```python
from build123d import *

# Parameters (mm, degrees)
EXTRUDE_THIN1_DEPTH             = 38.1
EXTRUDE1_DEPTH                  = 22.225
EXTRUDE2_REACH                  = 191.48
EXTRUDE2_END_RADIUS             = 58.254302176
SKETCH3_R                       = 14.2875
EXTRUDE2_DIRECTION_2_REACH      = 191.48
EXTRUDE2_DIRECTION_2_END_RADIUS = 36.120408138


with BuildPart() as part:
    # Sketch1 → Extrude-Thin1 (new, symmetric)
    with BuildSketch(Plane.XY):
        with BuildLine():
            Line((0, 0), (47.386965401, 0))
            ThreePointArc((47.386965401, 0), (51.527837673, 1.535887743), (53.665587121, 5.400574229))
            ThreePointArc((53.665587121, 5.400574229), (89.379977527, 36.120408138), (125.094367933, 5.400574229))
            ThreePointArc((125.094367933, 5.400574229), (127.232117381, 1.535887743), (131.372989653, 0))
            Line((131.372989653, 0), (178.759955054, 0))
            Line((178.759955054, 0), (178.759955054, -2.54))
            Line((178.759955054, -2.54), (131.372989653, -2.54))
            ThreePointArc((131.372989653, -2.54), (125.575768472, -0.38975716), (122.582919245, 5.02080392))
            ThreePointArc((122.582919245, 5.02080392), (89.379977527, 33.580408138), (56.177035809, 5.02080392))
            ThreePointArc((56.177035809, 5.02080392), (53.184186582, -0.38975716), (47.386965401, -2.54))
            Line((47.386965401, -2.54), (0, -2.54))
            Line((0, -2.54), (0, 0))
        make_face()
    extrude(amount=EXTRUDE_THIN1_DEPTH, both=True)



with BuildPart() as body_2:
    # Sketch2 → Extrude1 (new, symmetric)
    with BuildSketch(Plane.XY):
        with BuildLine():
            Line((69.175001958, 75.045019307), (109.584953096, 75.045019307))
            Line((109.584953096, 75.045019307), (109.584953096, 65.256940868))
            ThreePointArc((109.584953096, 65.256940868), (89.379977527, 61.640745213), (69.175001958, 65.256940868))
            Line((69.175001958, 65.256940868), (69.175001958, 75.045019307))
        make_face()
    extrude(amount=EXTRUDE1_DEPTH, both=True)


with BuildPart() as part_1:
    add(part.part)

    add(body_2.part)  # Extrude2 merges body 2
    # Extrude2: up to this cylinder (the profile starts outside it)
    extrude2_end = Plane(origin=(89.379977527, 119.89504739, 0), z_dir=(0, 0, -1)) * Cylinder(EXTRUDE2_END_RADIUS, 500.468604353, mode=Mode.PRIVATE)
    # Sketch3 → Extrude2 (add, up to the surface)
    with BuildSketch(Plane(origin=(0, 47.418237056, 0), x_dir=(-1, 0, 0), z_dir=(0, 1, 0)), mode=Mode.PRIVATE) as extrude2_sk1:
        with Locations(Location((-89.379977527, 0, 0), (0, 0, 270))):
            Circle(SKETCH3_R)
    extrude2_tool1 = extrude(extrude2_sk1.sketch, amount=EXTRUDE2_REACH, mode=Mode.PRIVATE) - extrude2_end
    add(extrude2_tool1.solids().sort_by_distance((89.379978, 47.418237, 0))[0])

    # Extrude2 direction 2: up to this cylinder (the profile starts outside it)
    extrude2_direction_2_end = Plane(origin=(89.379977527, 0, 0), z_dir=(0, 0, -1)) * Cylinder(EXTRUDE2_DIRECTION_2_END_RADIUS, 456.200816276, mode=Mode.PRIVATE)
    # Sketch3 → Extrude2 direction 2 (add, up to the surface)
    with BuildSketch(Plane(origin=(0, 47.418237056, 0), x_dir=(-1, 0, 0), z_dir=(0, 1, 0)), mode=Mode.PRIVATE) as extrude2_direction_2_sk1:
        with Locations(Location((-89.379977527, 0, 0), (0, 0, 270))):
            Circle(SKETCH3_R)
    extrude2_direction_2_tool1 = extrude(extrude2_direction_2_sk1.sketch, amount=-EXTRUDE2_DIRECTION_2_REACH, mode=Mode.PRIVATE) - extrude2_direction_2_end
    add(extrude2_direction_2_tool1.solids().sort_by_distance((89.379978, 47.418237, 0))[0])


solid = part_1.part
```
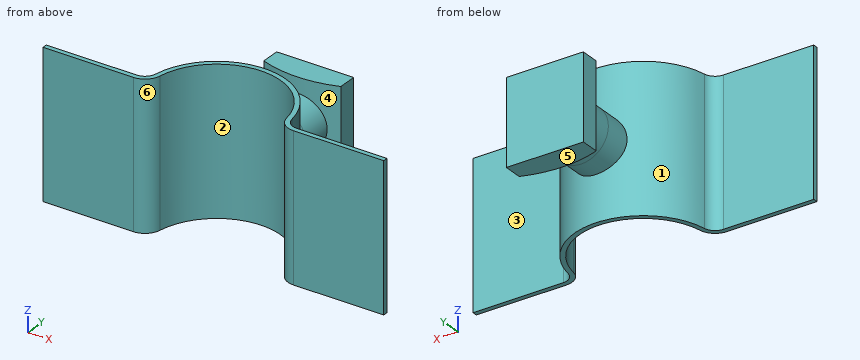
Model file for the job. Use its own axes, mm. Face numbers are marked on the shaded views. A direction names the side the tool comes from. Coordinates: 2 decimals unless noted, no trailing zeros. Write each loop counter-clockwise with the first axis right and the second up, starting at its lowest first coordinate (ties: lowest second). Pieces come first, ordered by that corner, then holes. Notation, with made-up numbers: (-8.5, 7) - (3.5, 7) arc R21 cw to (3.5, 15) - close; hole circle Ø8 at (34, -1.5). An arc over 180 degrees is marked (long way). One line per question, with ' | ' between items. Start each with the question number.
Q1. Cut at D-D, the plane x = 22.5. List the corners of the cut face in (y, z).
Q2. Cut at B-B, the plane z = 0. List the corners of the cut face in (x, y) (3 decimals).
Q3. Pin check, flat tips, straight feed: pin 1 (3 mm diameter, centred on y = 32.5, z = -29.5, fed in from +X); pin 2 (10 mm diameter, centred on y = 21.5, z = -12, fed in from -X); pin 3 (5 mm diameter, centred on x = 49, z = -22, fed in from -Y); pin 4 (5 mm diameter, centred on y = 28, z = -5.5, fed in from +X). Stop position of each tip, or through.
Q4. Cut at A-A, the plane y = 28. List the corners of the cut face in (x, z), then the cut area to 3 significant figures.
Q5. Pull direction X, two halves, no side cores. Call the marked faces 1, 2 and 3: pulls with the +X half, pulls with the -X half, needs draft (parallel to the pull), parting line crosses it, or undercut.
Q6. Drill centre lines: line 1 (Y direction, x = 33.5, z = 7); line 2 (X direction, y = 21, z = -5); line 3 (X direction, y = 70, z = 3) (3 decimals). Where is each one in solid material? Low to high. Write a range as [from, to].
Q7. 3-axis set-ups, long thin cutter, end or side, ignore diameter. For the marked faces 4, 5 and 6: which of +Z, -Z, +X, -X, +Y, -Y reach the whole face in a straight line?
Q8. Cut at C-C, the plane x = 106.5. List the corners of the cut face in (y, z) (3 decimals), then the cut area to 3 significant figures.
Answer below:
1) outline: (-2.54, -38.1) - (0, -38.1) - (0, 38.1) - (-2.54, 38.1) - close
2) outline: (0, -2.54) - (47.387, -2.54) arc R8.89 ccw to (56.177, 5.021) arc R33.58 cw to (122.583, 5.021) arc R8.89 ccw to (131.373, -2.54) - (178.76, -2.54) - (178.76, 0) - (131.373, 0) arc R6.35 cw to (125.094, 5.401) arc R36.12 ccw to (103.667, 33.175) - (103.667, 63.42) arc R58.254 ccw to (109.585, 65.257) - (109.585, 75.045) - (69.175, 75.045) - (69.175, 65.257) arc R58.254 ccw to (75.092, 63.42) - (75.092, 33.175) arc R36.12 ccw to (53.666, 5.401) arc R6.35 cw to (47.387, 0) - (0, 0) - close
3) pin 1: x = 107.92 | pin 2: x = 57.25 | pin 3: y = -2.54 | pin 4: x = 114.96
4) outline: (66.56, -38.1) - (70.84, -38.1) - (70.84, 38.1) - (66.56, 38.1) - close; (107.92, -38.1) - (112.2, -38.1) - (112.2, 38.1) - (107.92, 38.1) - close | area: 652 mm^2
5) face 1: parting line crosses it | face 2: undercut | face 3: needs draft
6) line 1: [-2.54, 0] | line 2: [59.99, 63.18], [115.58, 118.77] | line 3: [69.175, 109.585]
7) face 4: none | face 5: -Z, +X, -X, +Y | face 6: +Z, -Z, -Y
8) outline: (28.889, -38.1) - (31.805, -38.1) - (31.805, 38.1) - (28.889, 38.1) - close; (64.213, -22.225) - (75.045, -22.225) - (75.045, 22.225) - (64.213, 22.225) - close | area: 704 mm^2
